from build123d import *

# Parameters (mm, degrees)
SKETCH1_R           = 40
BOSS_EXTRUDE1_DEPTH = 2
SKETCH2_R           = 20
BOSS_EXTRUDE2_DEPTH = 10
CUT_EXTRUDE1_REACH  = 63.449
SKETCH3_R           = 2.073577671


with BuildPart() as part:
    # Sketch1 → Boss-Extrude1 (new body)
    with BuildSketch(Plane(origin=(0, 0, 0), x_dir=(1, 0, 0), z_dir=(0, 1, 0))):
        with Locations(Location((0, 0, 0), (0, 0, 270))):
            Circle(SKETCH1_R)
    boss_extrude1 = extrude(amount=BOSS_EXTRUDE1_DEPTH)

    # Sketch2 → Boss-Extrude2 (add)
    with BuildSketch(Plane(origin=(0, 2, 0), x_dir=(1, 0, 0), z_dir=(0, 1, 0))):
        with Locations(Location((0, 0, 0), (0, 0, 270))):
            Circle(SKETCH2_R)
    boss_extrude2 = extrude(amount=BOSS_EXTRUDE2_DEPTH)

    # Mirror1: Boss-Extrude1, Boss-Extrude2 across plane
    add(boss_extrude1.mirror(Plane.ZX.offset(12)))
    add(boss_extrude2.mirror(Plane.ZX.offset(12)))

    # Sketch3 → Cut-Extrude1 (cut, up to next)
    with BuildSketch(Plane.XZ, mode=Mode.PRIVATE) as cut_extrude1_sk1:
        with Locations(Location((0, 32.5, 0), (0, 0, 270))):
            Circle(SKETCH3_R)
    cut_extrude1_tool1 = extrude(cut_extrude1_sk1.sketch, amount=-CUT_EXTRUDE1_REACH, mode=Mode.PRIVATE) & part.part
    # Sketch3 → Cut-Extrude1 (cut, up to next)
    with BuildSketch(Plane.XZ, mode=Mode.PRIVATE) as cut_extrude1_sk2:
        with Locations(Location((32.5, 0, 0), (0, 0, 270))):
            Circle(SKETCH3_R)
    cut_extrude1_tool2 = extrude(cut_extrude1_sk2.sketch, amount=-CUT_EXTRUDE1_REACH, mode=Mode.PRIVATE) & part.part
    # Sketch3 → Cut-Extrude1 (cut, up to next)
    with BuildSketch(Plane.XZ, mode=Mode.PRIVATE) as cut_extrude1_sk3:
        with Locations(Location((0, -32.5, 0), (0, 0, 270))):
            Circle(SKETCH3_R)
    cut_extrude1_tool3 = extrude(cut_extrude1_sk3.sketch, amount=-CUT_EXTRUDE1_REACH, mode=Mode.PRIVATE) & part.part
    # Sketch3 → Cut-Extrude1 (cut, up to next)
    with BuildSketch(Plane.XZ, mode=Mode.PRIVATE) as cut_extrude1_sk4:
        with Locations(Location((-32.5, 0, 0), (0, 0, 270))):
            Circle(SKETCH3_R)
    cut_extrude1_tool4 = extrude(cut_extrude1_sk4.sketch, amount=-CUT_EXTRUDE1_REACH, mode=Mode.PRIVATE) & part.part
    add(cut_extrude1_tool1.solids().sort_by_distance((0, 0, 32.5))[0], mode=Mode.SUBTRACT)
    add(cut_extrude1_tool2.solids().sort_by_distance((32.5, 0, 0))[0], mode=Mode.SUBTRACT)
    add(cut_extrude1_tool3.solids().sort_by_distance((0, 0, -32.5))[0], mode=Mode.SUBTRACT)
    add(cut_extrude1_tool4.solids().sort_by_distance((-32.5, 0, 0))[0], mode=Mode.SUBTRACT)


solid = part.part
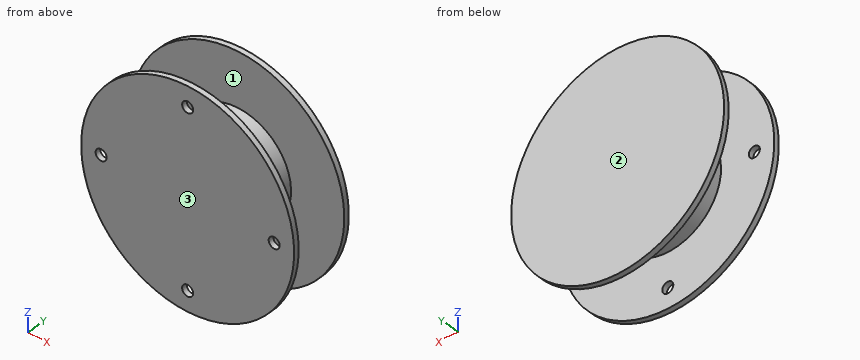
Build history of the part. All positions in model axes, mm. Face numbers are marked on the shaded views. Round coordinates to 2 decimals unless told otherwise and drop trailing zeros. Write each loop counter-clockwise with the first axis right and the second up, starting at its lowest first coordinate (ties: lowest second). Pieces come first, ordered by that corner, then holes. Notation, with made-up numbers: M -1.75,29.25 L 56.25,29.25 A20 ccw 56.25,54.25 Z; hole C 42,45.5 d5. An arc over 180 degrees is marked long. Use CSV: the item, a comma, the result in double quotes.
1. Saw through at B-B (z = 21.5). Give the cut face in (x, y).
Reply:
outline,"M -33.73,0 L 33.73,0 L 33.73,2 L -33.73,2 Z; M -33.73,22 L 33.73,22 L 33.73,24 L -33.73,24 Z"
2. Saw through at A-A (x = 0). Give the cut face in (y, z), plus the area to 3 significant figures.
Reply:
outline,"M 0,-40 L 2,-40 L 2,-34.57 L 0,-34.57 Z; M 0,-30.43 L 2,-30.43 L 2,-20 L 22,-20 L 22,-40 L 24,-40 L 24,40 L 22,40 L 22,20 L 2,20 L 2,30.43 L 0,30.43 Z; M 0,34.57 L 2,34.57 L 2,40 L 0,40 Z"
area,"1,100 mm²"
3. Saw through at D-D (x = 8). Give the cut face in (y, z), plus the area to 3 significant figures.
Reply:
outline,"M 0,-39.19 L 2,-39.19 L 2,-18.33 L 22,-18.33 L 22,-39.19 L 24,-39.19 L 24,39.19 L 22,39.19 L 22,18.33 L 2,18.33 L 2,39.19 L 0,39.19 Z"
area,"1,050 mm²"
4. Flat gauge pins, fed straight in: pin 1 (10 mm diameter, centred on x = -9.5, y = 21, fed in from +Z); pin 2 (10 mm diameter, centred on y = 10, z = 18, fed in from -X); pin 3 (3 mm diameter, centred on x = 6, y = 5.5, fed in from +Z). Where does each tip first touch, or does it go through?
Reply:
pin 1,"stops at z = 39.73"
pin 2,"stops at x = -15.2"
pin 3,"stops at z = 19.49"
5. Wall check: probe 1 along X at (y, z) = (1.4, 0); probe 2 along Y at (x, z) = (-23, -6.5); probe 3 along X at (y, z) = (0.4, 32.5). Give the ranges that are in metal, low to high. Write a range as from..to.
Reply:
probe 1,"x = -40..-34.57, -30.43..30.43, 34.57..40"
probe 2,"y = 0..2, 22..24"
probe 3,"x = -23.32..-2.07, 2.07..23.32"
6. Saw through at C-C (z = -32.5). Give the cut face in (x, y).
Reply:
outline,"M -23.32,0 L -2.07,0 L -2.07,2 L -23.32,2 Z; M -23.32,22 L 23.32,22 L 23.32,24 L -23.32,24 Z; M 2.07,0 L 23.32,0 L 23.32,2 L 2.07,2 Z"
7. Two-plate mould, pull along Y, no slides. Class the marked faces 1, 2 and 3: +Y half, -Y half, draft (parallel to the pull), parting line (faces both ways), or undercut.
Reply:
face 1,"undercut"
face 2,"+Y half"
face 3,"-Y half"
